```python
from build123d import *

# Parameters (mm, degrees)
SKETCH1_R           = 55.9705
SKETCH1_R_2         = 1.65
BOSS_EXTRUDE1_DEPTH = 3
SKETCH3_R           = 37.849999992
BOSS_EXTRUDE2_DEPTH = 2
BOSS_EXTRUDE2_TAPER = 2
CHAMFER1_SIZE       = 0.5
CHAMFER1_SIZE_2     = 0.518407978


with BuildPart() as part:
    # Sketch1 → Boss-Extrude1 (new body)
    with BuildSketch(Plane.XY):
        Circle(SKETCH1_R)
        with Locations((49.6705, 0)):
            Circle(SKETCH1_R_2, mode=Mode.SUBTRACT)
        with Locations((24.83525, 43.015914819)):
            Circle(SKETCH1_R_2, mode=Mode.SUBTRACT)
        with Locations((-24.83525, 43.015914819)):
            Circle(SKETCH1_R_2, mode=Mode.SUBTRACT)
        with Locations((-49.6705, 0)):
            Circle(SKETCH1_R_2, mode=Mode.SUBTRACT)
        with Locations((-24.83525, -43.015914819)):
            Circle(SKETCH1_R_2, mode=Mode.SUBTRACT)
        with Locations((24.83525, -43.015914819)):
            Circle(SKETCH1_R_2, mode=Mode.SUBTRACT)
    extrude(amount=BOSS_EXTRUDE1_DEPTH)

    # Sketch3 → Boss-Extrude2 (add)
    with BuildSketch(Plane(origin=(0, 0, 0), x_dir=(-1, 0, 0), z_dir=(0, 0, -1))):
        Circle(SKETCH3_R)
    extrude(amount=BOSS_EXTRUDE2_DEPTH, taper=BOSS_EXTRUDE2_TAPER)

    # Chamfer1
    # the kernel refuses this chamfer: 0.518407978, 0.5 mm, written as the material it takes off along each edge
    with BuildSketch(Plane(origin=(0, 0, -2), x_dir=(-1, 0, 0), z_dir=(0, 1, 0))) as chamfer1_piece_1:
        Polygon((37.780158453 + CHAMFER1_SIZE * 0.0348994967025, CHAMFER1_SIZE * 0.999390827019), (37.780158453 - CHAMFER1_SIZE_2, 0), (37.780158453, 0), align=None)
    revolve(axis=Axis((0, 0, -2), (0, 0, 1)), mode=Mode.SUBTRACT)


solid = part.part
```
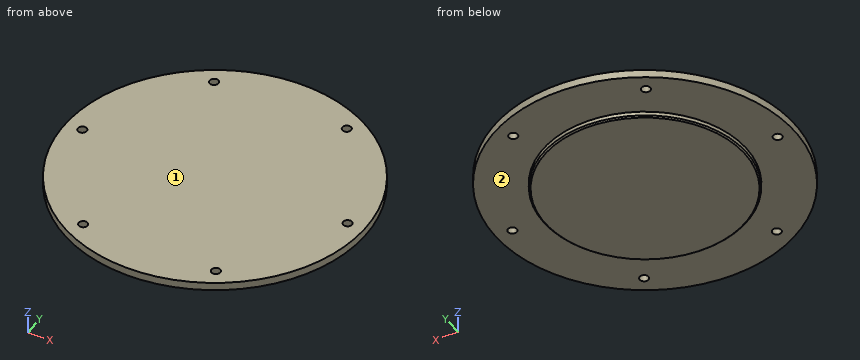
Can you work these out from the model? Positions are in its coordinate system, mm. Face numbers are marked on the shaded views. A direction names the side the tool comes from. Give positions to 0.01 mm unless a question says otherwise; leave off trailing zeros. Write each loop counter-clockwise with the first axis right and the second up, starting at its lowest first coordinate (ties: lowest second). Pieces come first, ordered by that corner, then holes. Notation, with made-up numbers: (87.25, 87.25) - (118.25, 87.25) arc R15 cw to (118.25, 95.25) - close; hole circle Ø5 at (-6.75, 76.5). An arc over 180 degrees is marked (long way). Write item = value, one per line. Start each with the question number.
1. Imagine slicing it at A-A (x = 0). Please give me the cut outline in (y, z), and give its area (3 significant figures).
2. Imagine slicing it at C-C (y = 0). Count the separate pieces of the cut face and the enclosed holes in it, and give its area (3 significant figures).
3. Imagine slicing it at D-D (x = -42.5). Please give me the cut outline in (y, z).
4. Please list where these lines run through material, in increasing order: line 1 (Y direction, x = -0.5, z = 0.3); line 2 (Z direction, x = -16.5, y = -51); line 3 (Y direction, x = 49.5, z = 0.7).
5. On a 3-axis mill with a long thin cutter (end or side, diameter ignored), from which of +Z, -Z, +X, -X, +Y, -Y can I reach the whole of each face in a straight line? I mean the marked faces 1 and 2. Say none if no direction works.
6. For pin 1 (4 mm diameter, centred on x = -35.5, y = 13.5, fed in from -Z); pin 2 (2 mm diameter, centred on x = -7.5, z = 1.5, fed in from +Y); pin 3 (2 mm diameter, centred on y = 2.5, z = 1.5, fed in from -X); pin 4 (5.5 mm diameter, centred on x = 49.67, y = 0, fed in from -Z), each with a flat end and sliding along its axis, tell me the tip position at first contact or that it passes through.
7. Imagine slicing it at B-B (z = 2). Please give me the cut outline in (x, y).
Worked answers:
q1.outline = (-55.97, 0) - (-37.85, 0) - (-37.8, -1.5) - (-37.26, -2) - (37.26, -2) - (37.8, -1.5) - (37.85, 0) - (55.97, 0) - (55.97, 3) - (-55.97, 3) - close
q1.area = 487 mm2
q2.separate_pieces = 3
q2.enclosed_holes = 0
q2.area = 467 mm2
q3.outline = (-36.42, 0) - (36.42, 0) - (36.42, 3) - (-36.42, 3) - close
q4.line_1 = -55.97 to 55.97
q4.line_2 = 0 to 3
q4.line_3 = -26.12 to -1.64, 1.64 to 26.12
q5.face_1 = +Z, +X, -X, +Y, -Y
q5.face_2 = -Z
q6.pin_1 = -2
q6.pin_2 = 55.59
q6.pin_3 = -55.95
q6.pin_4 = 0
q7.outline = circle Ø111.94 at (0, 0); hole circle Ø3.3 at (-49.67, 0); hole circle Ø3.3 at (-24.84, -43.02); hole circle Ø3.3 at (-24.84, 43.02); hole circle Ø3.3 at (24.84, -43.02); hole circle Ø3.3 at (24.84, 43.02); hole circle Ø3.3 at (49.67, 0)
